from build123d import *

# Parameters (mm, degrees)
BOSS_EXTRUDE2_DEPTH  = 1.5
SKETCH1_4_W          = 10
SKETCH1_4_H          = 7
BOSS_EXTRUDE3_DEPTH  = 1.5
SKETCH1_14_W         = 2
SKETCH1_14_H         = 20.5
BOSS_EXTRUDE11_DEPTH = 5
SKETCH1_16_W         = 1.5
SKETCH1_16_H         = 25
BOSS_EXTRUDE12_DEPTH = 11.6
SKETCH2_W            = 15.3
SKETCH2_H            = 25
BOSS_EXTRUDE13_DEPTH = 1.5


with BuildPart() as part:
    # Sketch1 → Boss-Extrude2 (new body)
    with BuildSketch(Plane(origin=(0, 0, 0), x_dir=(1, 0, 0), z_dir=(0, 1, 0))):
        Polygon((49.5, 70), (-4.5, 70), (-4.5, 49.5), (-6.5, 49.5), (-6.5, 42.5), (-6.5, 12.5), (-6.5, 5.5), (-4.5, 5.5), (-4.5, -15), (21.3, -15), (32.3, -15), (47.433426619, -15), (49.5, -15), (49.5, 10), (51, 10), (51, -15), (52.3, -15), (53.8, -15), (59.19614989, -15), (63.3, -15), (63.3, 10), (64.8, 10), (64.8, 11.5), (64.8, 45), (63.3, 45), (63.3, 70), (60.5, 70), (51, 70), (51, 45), (49.5, 45), align=None)
    extrude(amount=BOSS_EXTRUDE2_DEPTH)

    # Sketch1<4> → Boss-Extrude3 (add)
    with BuildSketch(Plane(origin=(0, 0, 0), x_dir=(1, 0, 0), z_dir=(0, 1, 0))):
        with Locations((-11.5, 46)):
            Rectangle(SKETCH1_4_W, SKETCH1_4_H)
        with Locations((-11.5, 9)):
            Rectangle(SKETCH1_4_W, SKETCH1_4_H)
    extrude(amount=BOSS_EXTRUDE3_DEPTH)

    # Sketch1<14> → Boss-Extrude11 (add)
    with BuildSketch(Plane(origin=(0, 0, 0), x_dir=(1, 0, 0), z_dir=(0, 1, 0))):
        with Locations((-5.5, 59.75)):
            Rectangle(SKETCH1_14_W, SKETCH1_14_H)
        with Locations((-5.5, -4.75)):
            Rectangle(SKETCH1_14_W, SKETCH1_14_H)
    extrude(amount=BOSS_EXTRUDE11_DEPTH)

    # Sketch1<16> → Boss-Extrude12 (add)
    with BuildSketch(Plane(origin=(0, 0, 0), x_dir=(1, 0, 0), z_dir=(0, 1, 0))):
        with Locations((50.25, -2.5)):
            Rectangle(SKETCH1_16_W, SKETCH1_16_H)
        with Locations((64.05, -2.5)):
            Rectangle(SKETCH1_16_W, SKETCH1_16_H)
        with Locations((64.05, 57.5)):
            Rectangle(SKETCH1_16_W, SKETCH1_16_H)
        with Locations((50.25, 57.5)):
            Rectangle(SKETCH1_16_W, SKETCH1_16_H)
    extrude(amount=BOSS_EXTRUDE12_DEPTH)

    # Sketch2 → Boss-Extrude13 (add)
    with BuildSketch(Plane(origin=(0, 11.6, 0), x_dir=(1, 0, 0), z_dir=(0, 1, 0))):
        with Locations((57.15, 57.5)):
            Rectangle(SKETCH2_W, SKETCH2_H)
        with Locations((57.15, -2.5)):
            Rectangle(SKETCH2_W, SKETCH2_H)
    extrude(amount=BOSS_EXTRUDE13_DEPTH)


solid = part.part
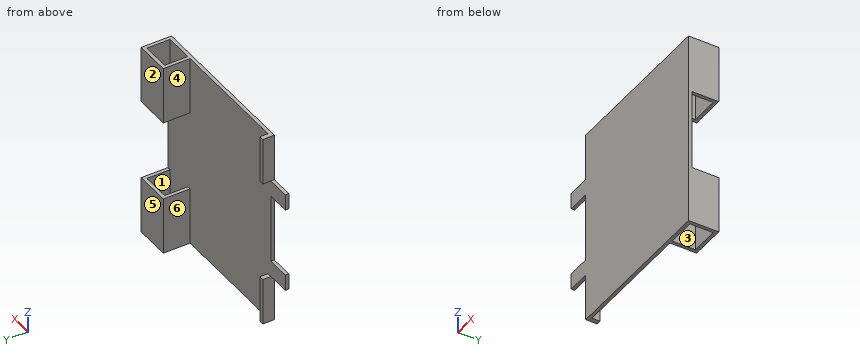
The model under review builds one solid part; all positions refer to its coordinate system, in mm. Face numbers are marked on the shaded views. A direction names the side the tool comes from. Give positions to 0.01 mm unless a question says otherwise; leave off trailing zeros. Order: outer loops, then holes, each group sorted by start corner. A loop starts at its lowest first (then second) coordinate and runs counter-clockwise, first axis right, second up. Notation, with made-up numbers: M 46,74 L 86,74 A21 cw 86,100 Z; hole C 34.5,52 d1. An arc over 180 degrees is marked long. Answer in a Markdown table with one row per item. Add a question column.
1. Mouldability with a two-part tool opening along Y and no side actions: class the marked faces 1, 2, 3 and 4 as released by +Y, released by -Y, zero draft, split by the parting line, or undercut.
2. Add section C-C on y = 10.25. State the section outline as (x, z) points, plus the area to 3 significant figures.
3. To check wall thickness, follow line 1 along X through (y, z) = (2.75, 7); line 2 along X through (y, z) = (9.25, -54.5); line 3 along Y through (x, z) = (52.5, -6). State the ranges of each line that lie inside material, in increasing order.
4. Machinability: for the marked faces 5 and 6, which of the approach directions +Z, -Z, +X, -X, +Y, -Y give a long, thin tool a straight path to every point of the face, cutting with its end or side? Answer none if there is none.
5. For pin 1 Ø5 at (x, z) = (-5.5, -52.5) entering from +Y; pin 2 Ø0.8 at (y, z) = (1, -32.5) entering from -X; pin 3 Ø3 at (x, z) = (3, -19.5) entering from +Y, all flat-tipped, find the tip position at first contact; note any pin that passes through.
6. Add section B-B on x = 54. State the section outline as (y, z) points.
7. Add section D-D on z = -54. State the section outline as (x, y) points, plus the area to 3 significant figures.
8. Add section A-A on x = -12. State the section outline as (y, z) points.
The answers:
| question | item | result |
|---|---|---|
| 1 | face 1 | undercut |
| 1 | face 2 | released by +Y |
| 1 | face 3 | undercut |
| 1 | face 4 | zero draft |
| 2 | outline | M 49.5,-70 L 51,-70 L 51,-45 L 49.5,-45 Z; M 49.5,-10 L 51,-10 L 51,15 L 49.5,15 Z; M 63.3,-70 L 64.8,-70 L 64.8,-45 L 63.3,-45 Z; M 63.3,-10 L 64.8,-10 L 64.8,15 L 63.3,15 Z |
| 2 | area | 150 mm2 |
| 3 | line 1 | -6.5 to -4.5, 49.5 to 51, 63.3 to 64.8 |
| 3 | line 2 | 49.5 to 51, 63.3 to 64.8 |
| 3 | line 3 | 0 to 1.5, 11.6 to 13.1 |
| 4 | face 5 | +Z, -Z, +X, -X, +Y |
| 4 | face 6 | +Z, -Z, +Y |
| 5 | pin 1 | y = 5 |
| 5 | pin 2 | x = -6.5 |
| 5 | pin 3 | y = 1.5 |
| 6 | outline | M 0,-70 L 1.5,-70 L 1.5,15 L 0,15 Z; M 11.6,-70 L 13.1,-70 L 13.1,-45 L 11.6,-45 Z; M 11.6,-10 L 13.1,-10 L 13.1,15 L 11.6,15 Z |
| 7 | outline | M -6.5,0 L 64.8,0 L 64.8,13.1 L 49.5,13.1 L 49.5,1.5 L -4.5,1.5 L -4.5,5 L -6.5,5 Z; hole M 51,1.5 L 63.3,1.5 L 63.3,11.6 L 51,11.6 Z |
| 7 | area | 167 mm2 |
| 8 | outline | M 0,-49.5 L 1.5,-49.5 L 1.5,-42.5 L 0,-42.5 Z; M 0,-12.5 L 1.5,-12.5 L 1.5,-5.5 L 0,-5.5 Z |
